```python
from build123d import *

# Parameters (mm, degrees)
SKETCH1_R           = 2.5
BOSS_EXTRUDE1_DEPTH = 3
SKETCH2_R           = 1.5
CUT_EXTRUDE1_DEPTH  = 77.127156728
FILLET1_R           = 10


with BuildPart() as part:
    # Sketch1 → Boss-Extrude1 (new body)
    with BuildSketch(Plane.XY):
        with BuildLine():
            Line((0, -19), (30, -19))
            Line((30, -19), (64.201367261, 15.201367261))
            Line((64.201367261, 15.201367261), (58.615223689, 20.787510832))
            Line((58.615223689, 20.787510832), (31.745166004, -6.082546853))
            Line((31.745166004, -6.082546853), (17.320187668, 8.342431483))
            Line((17.320187668, 8.342431483), (44.190245353, 35.212489168))
            Line((44.190245353, 35.212489168), (38.604101782, 40.798632739))
            Line((38.604101782, 40.798632739), (16.805469042, 19))
            Line((16.805469042, 19), (0, 19))
            ThreePointArc((0, 19), (-19, 0), (0, -19))
        make_face()
        Circle(SKETCH1_R, mode=Mode.SUBTRACT)
    extrude(amount=BOSS_EXTRUDE1_DEPTH)

    # Sketch2 → Cut-Extrude1 (cut, through all)
    with BuildSketch(Plane.XY.offset(3)):
        with Locations((38.878105659, 35.574881393)):
            Circle(SKETCH2_R)
        with Locations((58.977615915, 15.475371138)):
            Circle(SKETCH2_R)
    extrude(amount=-CUT_EXTRUDE1_DEPTH, mode=Mode.SUBTRACT)

    # Fillet1
    fillet1_edges = [part.edges().sort_by_distance(p)[0] for p in [
        (30, -19, 1.5),
        (16.805469042, 19, 1.5),
    ]]
    fillet(fillet1_edges, radius=FILLET1_R)


solid = part.part
```
Design review of the part built by this model. Coordinates are the model's own, in mm. A direction names the side the tool comes from. Give positions to 0.01 mm unless a question says otherwise; leave off trailing zeros. Order: outer loops, then holes, each group sorted by start corner. A loop starts at its lowest first (then second) coordinate and runs counter-clockwise, first axis right, second up. Notation, with made-up numbers: (12, 0) - (51, 0) arc R16 cw to (51, 26) - close; hole circle Ø5 at (59.5, -35). An arc over 180 degrees is marked (long way). Use a Markdown table: item, result. Add a question column.
(1) Add section D-D on y = 4.5. Give the boundary of the cut face in (x, z).
(2) Clearance check with flat-ended pins moving along their axes: P1, Ø1, axis at y = -12, z = 2.5, coming from the -X side; P2, Ø1, axis at y = -12.5, z = 2, coming from the +X side; P3, Ø4.5, axis at x = 0, y = 0, coming from the +Z side; P4, Ø0.9, axis at x = 8, z = 1.5, coming from the +Y side. State where each tip first meets the part, or that it passes through.
(3) Mouldability with a two-part tool opening along X and no side actions: class faces 3 (the face through (6, 19, 1)), 4 (the face through (57.48, 15.54, 1.52)), 5 (the face through (29.301, 31.496, 1.479)) as +X half, -X half, draft (parallel to the pull), parting line (faces both ways), or undercut.
(4) Add section A-A on x = 21. Give the boundary of the cut face in (y, z).
(5) Add section C-C on z = 1.75. Give the boundary of the cut face in (x, y), then the cut area to 3 significant figures.
(6) Wall thickness on probe 1 along Y at (x, z) = (0, 2); probe 2 along Y at (x, z) = (39.5, 0.8); probe 3 along X at (y, z) = (8.5, 2.1): over which ranges is each line inside the solid? List them lowest first. Write a range as [from, to].
(7) Machinability: for faces 1 (the face through (13, 5, 3)), 2 (the face through (30.57, 21.59, 1.48)), which of the approach directions +Z, -Z, +X, -X, +Y, -Y give a long, thin tool a straight path to every point of the face, cutting with its end or side? Answer none if there is none.
(8) Add section B-B on y = -1.5. Give the boundary of the cut face in (x, z), then the cut area to 3 significant figures.
Report:
| question | item | result |
|---|---|---|
| 1 | outline | (-18.46, 0) - (21.16, 0) - (21.16, 3) - (-18.46, 3) - close; (42.33, 0) - (53.5, 0) - (53.5, 3) - (42.33, 3) - close |
| 2 | P1 | stops at x = -15.12 |
| 2 | P2 | stops at x = 37 |
| 2 | P3 | passes through |
| 2 | P4 | stops at y = 19 |
| 3 | face 3 | draft |
| 3 | face 4 | undercut |
| 3 | face 5 | -X half |
| 4 | outline | (-19, 0) - (4.66, 0) - (4.66, 3) - (-19, 3) - close; (12.02, 0) - (23.19, 0) - (23.19, 3) - (12.02, 3) - close |
| 5 | outline | (0, -19) - (25.86, -19) arc R10 ccw to (32.93, -16.07) - (64.2, 15.2) - (58.62, 20.79) - (31.75, -6.08) - (17.32, 8.34) - (44.19, 35.21) - (38.6, 40.8) - (19.73, 21.93) arc R10 cw to (12.66, 19) - (0, 19) arc R19 ccw to start; hole circle Ø5 at (0, 0); hole circle Ø3 at (38.88, 35.57); hole circle Ø3 at (58.98, 15.48) |
| 5 | area | 2,080 mm² |
| 6 | probe 1 | y = [-19, -2.5], [2.5, 19] |
| 6 | probe 2 | y = [-9.5, 1.67], [30.52, 34.21], [36.94, 39.9] |
| 6 | probe 3 | x = [-16.99, 17.48], [46.33, 57.5] |
| 7 | face 1 | +Z, +X, -X, +Y, -Y |
| 7 | face 2 | +Z, -Z |
| 8 | outline | (-18.94, 0) - (-2, 0) - (-2, 3) - (-18.94, 3) - close; (2, 0) - (27.16, 0) - (27.16, 3) - (2, 3) - close; (36.33, 0) - (47.5, 0) - (47.5, 3) - (36.33, 3) - close |
| 8 | area | 160 mm² |
